Part model, mm, in its own coordinate system. A direction names the side the tool comes from. Give positions to 0.01 mm unless a question says otherwise; leave off trailing zeros. Loops run counter-clockwise (first coordinate to the right, second up) from the corner with the lowest first, then second, coordinate; pieces in that order, holes last. Notation, with made-up numbers: M -26.5,19.25 L 17.5,19.25 A28 cw 17.5,42.25 Z; hole C 4,67.25 d8. An arc over 180 degrees is marked long. Answer in a Markdown table with one row per item.
from build123d import *

# Parameters (mm, degrees)
CROQUIS2_R              = 2
CROQUIS2_W              = 20.3
CROQUIS2_H              = 40.3
SALIENTE_EXTRUIR2_DEPTH = 3


with BuildPart() as part:
    # Croquis2 → Saliente-Extruir2 (new body)
    with BuildSketch(Plane.XY):
        with BuildLine():
            Line((54.85, 71.478027684), (54.85, 8.521972316))
            ThreePointArc((54.85, 8.521972316), (49.890052554, 0.594274169), (41.065374433, -2.5))
            Line((41.065374433, -2.5), (13, -2.5))
            Line((13, -2.5), (13, -17.5))
            Line((13, -17.5), (41.065374433, -17.5))
            ThreePointArc((41.065374433, -17.5), (41.786840737, -15.033246538), (42.220486043, -12.5))
            Line((42.220486043, -12.5), (67.5, -12.5))
            Line((67.5, -12.5), (72.5, -12.5))
            Line((72.5, -12.5), (97.779513957, -12.5))
            ThreePointArc((97.779513957, -12.5), (98.213159263, -15.033246538), (98.934625567, -17.5))
            Line((98.934625567, -17.5), (127, -17.5))
            Line((127, -17.5), (127, -2.5))
            Line((127, -2.5), (98.934625567, -2.5))
            ThreePointArc((98.934625567, -2.5), (90.109947446, 0.594274169), (85.15, 8.521972316))
            Line((85.15, 8.521972316), (85.15, 71.478027684))
            ThreePointArc((85.15, 71.478027684), (90.109947446, 79.405725831), (98.934625567, 82.5))
            Line((98.934625567, 82.5), (127, 82.5))
            Line((127, 82.5), (127, 97.5))
            Line((127, 97.5), (98.934625567, 97.5))
            ThreePointArc((98.934625567, 97.5), (98.213159263, 95.033246538), (97.779513957, 92.5))
            Line((97.779513957, 92.5), (72.5, 92.5))
            Line((72.5, 92.5), (67.5, 92.5))
            Line((67.5, 92.5), (42.220486043, 92.5))
            ThreePointArc((42.220486043, 92.5), (41.786840737, 95.033246538), (41.065374433, 97.5))
            Line((41.065374433, 97.5), (13, 97.5))
            Line((13, 97.5), (13, 82.5))
            Line((13, 82.5), (41.065374433, 82.5))
            ThreePointArc((41.065374433, 82.5), (49.890052554, 79.405725831), (54.85, 71.478027684))
        make_face()
        with Locations((65, 64.15)):
            Circle(CROQUIS2_R, mode=Mode.SUBTRACT)
        with Locations(Location((75, 64.15, 0), (0, 0, 180))):
            Circle(CROQUIS2_R, mode=Mode.SUBTRACT)
        with Locations((75, 15.85)):
            Circle(CROQUIS2_R, mode=Mode.SUBTRACT)
        with Locations(Location((65, 15.85, 0), (0, 0, 180))):
            Circle(CROQUIS2_R, mode=Mode.SUBTRACT)
        with Locations((20, -10)):
            Circle(CROQUIS2_R, mode=Mode.SUBTRACT)
        with Locations(Location((120, -10, 0), (0, 0, 180))):
            Circle(CROQUIS2_R, mode=Mode.SUBTRACT)
        with Locations((120, 90)):
            Circle(CROQUIS2_R, mode=Mode.SUBTRACT)
        with Locations(Location((20, 90, 0), (0, 0, 180))):
            Circle(CROQUIS2_R, mode=Mode.SUBTRACT)
        with Locations((70, 40)):
            Rectangle(CROQUIS2_W, CROQUIS2_H, mode=Mode.SUBTRACT)
    extrude(amount=SALIENTE_EXTRUIR2_DEPTH)


solid = part.part
(1) Pin check, flat tips, straight feed: pin 1 Ø0.9 at (y, z) = (44.5, 1.5) entering from -X; pin 2 Ø6.5 at (x, y) = (65, 64.15) entering from -Z; pin 3 Ø0.9 at (x, z) = (71, 2) entering from +Y; pin 4 Ø1.5 at (y, z) = (49.5, 1) entering from +X. Stop position of each tip, or through.
Recorded:
| item | result |
|---|---|
| pin 1 | stops at x = 54.85 |
| pin 2 | stops at z = 0 |
| pin 3 | stops at y = 92.5 |
| pin 4 | stops at x = 85.15 |
(2) Saw through at A-A (y = 46). Write the cut outline in (x, z), plus the area to 3 significant figures.
Recorded:
| item | result |
|---|---|
| outline | M 54.85,0 L 59.85,0 L 59.85,3 L 54.85,3 Z; M 80.15,0 L 85.15,0 L 85.15,3 L 80.15,3 Z |
| area | 30.0 mm^2 |
(3) Saw through at B-B (x = 120). Write the cut outline in (y, z).
Recorded:
| item | result |
|---|---|
| outline | M -17.5,0 L -12,0 L -12,3 L -17.5,3 Z; M -8,0 L -2.5,0 L -2.5,3 L -8,3 Z; M 82.5,0 L 88,0 L 88,3 L 82.5,3 Z; M 92,0 L 97.5,0 L 97.5,3 L 92,3 Z |
(4) Pull direction Y, two halves, no side cores. Call faces 6 (the face through (127, -10, 1)), 7 (the face through (98.22, 95.07, 1.48)), 8 (the face through (85.15, 40, 1)): +Y half, -Y half, draft (parallel to the pull), parting line (faces both ways), or undercut.
Recorded:
| item | result |
|---|---|
| face 6 | draft |
| face 7 | +Y half |
| face 8 | undercut |
(5) Drill centre lines: line 1 along Y through (x, z) = (65, 1.5); line 2 along Y through (x, z) = (120, 2.3); line 3 along Y through (x, z) = (30, 0.2). Where is each one in solid material? Low to high.
Recorded:
| item | result |
|---|---|
| line 1 | y = -12.5 to 13.85, 17.85 to 19.85, 60.15 to 62.15, 66.15 to 92.5 |
| line 2 | y = -17.5 to -12, -8 to -2.5, 82.5 to 88, 92 to 97.5 |
| line 3 | y = -17.5 to -2.5, 82.5 to 97.5 |
(6) Which spindle directions (+Z, -Z, +X, -X, +Y, -Y) get a long thin tool onto all of the face, cutting with end or side? Do faces 1 (the face through (41.78, -15.07, 1.48)), 2 (the face through (54.85, 40, 1)), 3 (the face through (13, -10, 1)), 4 (the face through (113, -17.5, 1)), 5 (the face through (90.215, 0.511, 1.479)). Say none if no direction does.
Recorded:
| item | result |
|---|---|
| face 1 | +Z, -Z, -Y |
| face 2 | +Z, -Z, -X |
| face 3 | +Z, -Z, -X, +Y, -Y |
| face 4 | +Z, -Z, +X, -X, -Y |
| face 5 | +Z, -Z, +X |
(7) Saw through at D-D (x = 53). Write the cut outline in (y, z).
Recorded:
| item | result |
|---|---|
| outline | M -12.5,0 L 4.06,0 L 4.06,3 L -12.5,3 Z; M 75.94,0 L 92.5,0 L 92.5,3 L 75.94,3 Z |
(8) Saw through at C-C (y = 64.15). Write the cut outline in (x, z).
Recorded:
| item | result |
|---|---|
| outline | M 54.85,0 L 63,0 L 63,3 L 54.85,3 Z; M 67,0 L 73,0 L 73,3 L 67,3 Z; M 77,0 L 85.15,0 L 85.15,3 L 77,3 Z |
